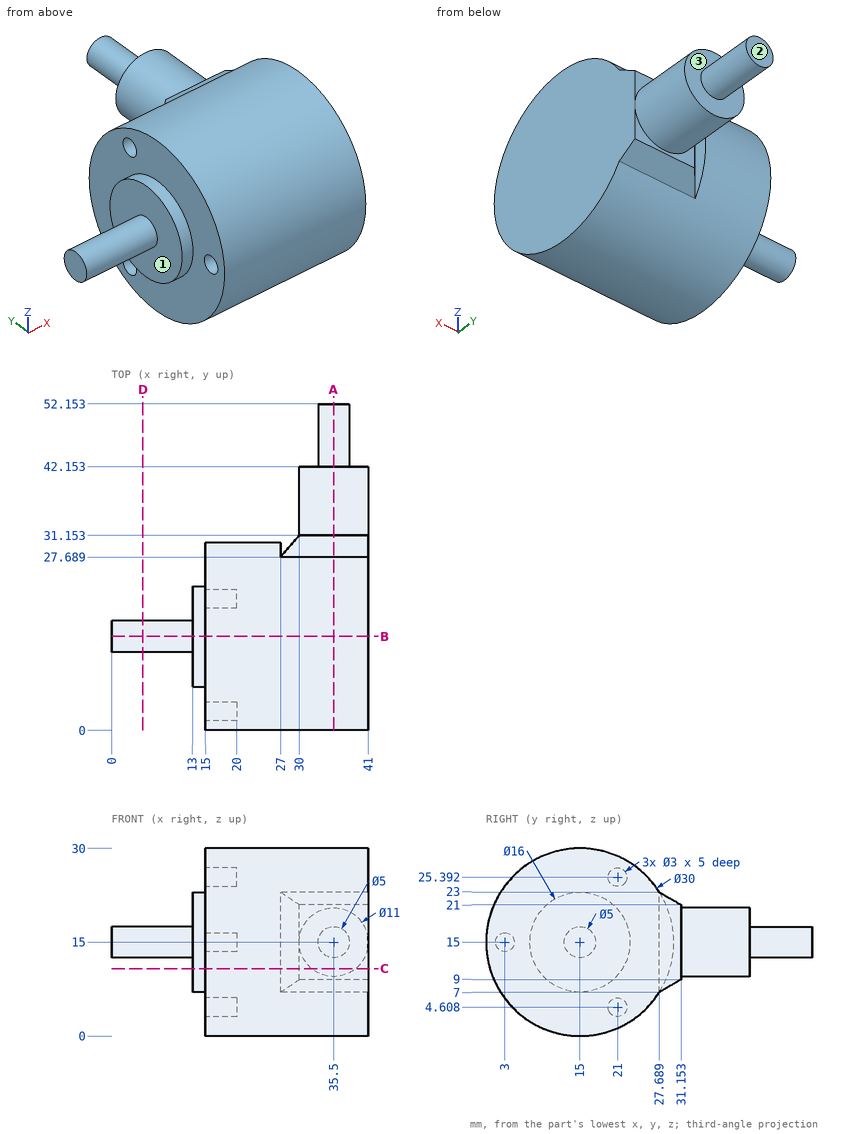
Verification items for this drawing (mm, ordinates from the low corner). A direction names the side the tool comes from. Round coordinates to 2 decimals unless told otherwise and drop trailing zeros. Order: outer loops, then holes, each group sorted by start corner. A loop starts at its lowest first (then second) coordinate and runs counter-clockwise, first axis right, second up. Notation, with made-up numbers: M -10.75,-18.5 L 41.25,-18.5 A13 cw 41.25,-2.5 Z; hole C 54.25,58.25 d5. An arc over 180 degrees is marked long. Answer in a Markdown table with one row per item. Add a question column.
Item 1: Depth check by flat-ended pin: pin 1 Ø3 at (x, z) = (24, 12) entering from +Y (1 decimal); pin 2 Ø6 at (x, y) = (28, 40) entering from +Z; pin 3 Ø9 at (y, z) = (20, 9.5) entering from -X. Enter the tip coordinate at first touch or a pass-through.
Item 2: Sectioned sample at A-A, the plane x = 35.5. Enter the section's corners in (y, z).
Item 3: Sectioned sample at C-C, the plane z = 10.75. Enter the section's corners in (x, y) (1 decimal).
Item 4: Set-up check for the marked faces 1, 2 and 3: record each of +Z, -Z, +X, -X, +Y, -Y from which the full face is reachable in a straight line by a thin tool's end or side.
Item 5: Material ranges on L1, parallel to Y at x = 17, z = 15; L2, parallel to X at y = 6, z = 13.5; L3, parallel to Y at x = 27.5, z = 24.25, recorded low to high. Write a range as [from, to].
Item 6: Sectioned sample at B-B, the plane y = 15. Enter the section's corners in (x, z).
Item 7: Sectioned sample at D-D, the plane x = 5. Enter the section's corners in (y, z).
Filled in:
| question | item | result |
|---|---|---|
| 1 | pin 1 | stops at y = 29.9 |
| 1 | pin 2 | stops at z = 18.16 |
| 1 | pin 3 | stops at x = 13 |
| 2 | outline | M 27.69,7 L 31.15,9 L 31.15,9.5 L 42.15,9.5 L 42.15,12.5 L 52.15,12.5 L 52.15,17.5 L 42.15,17.5 L 42.15,20.5 L 31.15,20.5 L 31.15,21 L 27.69,23 A15 ccw long Z |
| 3 | outline | M 13,8.2 L 15,8.2 L 15,0.6 L 41,0.6 L 41,31.2 L 39,31.2 L 39,42.2 L 32,42.2 L 32,31.2 L 30,31.2 L 27,27.7 L 27,29.4 L 15,29.4 L 15,21.8 L 13,21.8 Z |
| 4 | face 1 | -X |
| 4 | face 2 | +Z, -Z, +X, -X, +Y |
| 4 | face 3 | +Y |
| 5 | L1 | y = [0, 1.5], [4.5, 30] |
| 5 | L2 | x = [15, 41] |
| 5 | L3 | y = [3.19, 26.81] |
| 6 | outline | M 0,12.5 L 13,12.5 L 13,7 L 15,7 L 15,0 L 41,0 L 41,30 L 15,30 L 15,23 L 13,23 L 13,17.5 L 0,17.5 Z |
| 7 | outline | C 15,15 d5 |
